Geometry: final body of the model. Coordinates: model frame, mm. Give positions to 0.01 mm unless a question says otherwise; leave off trailing zeros. Write each loop counter-clockwise with the first axis right and the second up, starting at its lowest first coordinate (ties: lowest second). Pieces come first, ordered by that corner, then holes. Notation, with made-up numbers: M -20,78 L 7,78 A35 ccw 7,114 Z; hole C 14,8.5 d11. An arc over 180 degrees is marked long. Use a Markdown table: item, result. Add a question column.
(1) Cut plane D-D (x = 0). Output: boundary loops of the cut face in (y, z) (3 decimals), plus the area to 3 significant figures.
(2) Material intervals for L1, parallel to X at y = -0.5, z = 4.25; L2, parallel to X at y = 5, z = 0.75; L3, parallel to X at y = -12, z = 4.75, sorted ascending.
(3) Cut plane A-A (x = -30.48). Output: boundary loops of the cut face in (y, z) (3 decimals), plus the area to 3 significant figures.
(4) Draft query along Y for faces 1 (the cylindrical face through (0.13, 15.11, 3.46)), 2 (the cylindrical face through (-45.713, 0.47, 3.461)), 3 (the cylindrical face through (19.98, 3.31, 3.44)), 4 (the cylindrical face through (-15.262, -10.234, 3.461)). Return one class per face: released by +Y, released by -Y, zero draft, split by the parting line, or undercut.
(5) Cut plane B-B (z = 3.75). Output: boundary loops of the cut face in (x, y) (3 decimals), plus the area to 3 significant figures.
(6) Cut plane C-C (y = -5). State how many separate pieces and enclosed holes the cut face has, plus the area to 3 significant figures.
(7) Pin query (flat end, axial travel): pin 1 Ø1 at (x, z) = (-11, 4) entering from -Y; pin 2 Ø1.5 at (x, z) = (-6, 4.5) entering from -Y. Return the tip coordinate at first contact, or that it passes through.
```python
from build123d import *

# Parameters (mm, degrees)
F0_R     = 11.0109
F1_DEPTH = 6.985
F2_SIZE  = 1.27
F3_SIZE  = 1.27


with BuildPart() as f1:
    # F0 (on Top) → F1 (new body)
    with BuildSketch(Plane.XY):
        with BuildLine():
            Line((15.1104870251, 0), (11.0109, 0))
            ThreePointArc((11.0109, 0), (0, -11.0109), (-11.0109, 0))
            Line((-11.0109, 0), (-15.1104870251, 0))
            ThreePointArc((-15.1104870251, 0), (-13.4476229912, -6.8911721805), (-8.8250173454, -12.2656384664))
            ThreePointArc((-8.8250173454, -12.2656384664), (0, -15.1104870251), (8.8250173454, -12.2656384664))
            ThreePointArc((8.8250173454, -12.2656384664), (13.4476229912, -6.8911721805), (15.1104870251, 0))
        make_face()
        with BuildLine():
            ThreePointArc((-11.0109, 0), (0, 11.0109), (11.0109, 0))
            Line((11.0109, 0), (15.1104870251, 0))
            ThreePointArc((15.1104870251, 0), (13.4476229912, 6.8911721805), (8.8250173454, 12.2656384664))
            ThreePointArc((8.8250173454, 12.2656384664), (0, 15.1104870251), (-8.8250173454, 12.2656384664))
            ThreePointArc((-8.8250173454, 12.2656384664), (-13.4476229912, 6.8911721805), (-15.1104870251, 0))
            Line((-15.1104870251, 0), (-11.0109, 0))
        make_face()
        with BuildLine():
            ThreePointArc((8.8250173454, 12.2656384664), (13.4476229912, 6.8911721805), (15.1104870251, 0))
            Line((15.1104870251, 0), (15.24, 0))
            ThreePointArc((15.24, 0), (16.8932840155, 6.9035316148), (21.4944289707, 12.3092287848))
            ThreePointArc((21.4944289707, 12.3092287848), (15.1667904983, 10.2333297341), (8.8250173454, 12.2656384664))
        make_face()
        with BuildLine():
            Line((15.24, 0), (15.1104870251, 0))
            ThreePointArc((15.1104870251, 0), (13.4476229912, -6.8911721805), (8.8250173454, -12.2656384664))
            ThreePointArc((8.8250173454, -12.2656384664), (15.1667904983, -10.2333297341), (21.4944289707, -12.3092287848))
            ThreePointArc((21.4944289707, -12.3092287848), (16.8932840155, -6.9035316148), (15.24, 0))
        make_face()
        with BuildLine():
            ThreePointArc((-8.8250173454, -12.2656384664), (-13.4476229912, -6.8911721805), (-15.1104870251, 0))
            Line((-15.1104870251, 0), (-15.24, 0))
            ThreePointArc((-15.24, 0), (-16.8932840155, -6.9035316148), (-21.4944289707, -12.3092287848))
            ThreePointArc((-21.4944289707, -12.3092287848), (-15.1667904983, -10.2333297341), (-8.8250173454, -12.2656384664))
        make_face()
        with BuildLine():
            Line((-15.24, 0), (-15.1104870251, 0))
            ThreePointArc((-15.1104870251, 0), (-13.4476229912, 6.8911721805), (-8.8250173454, 12.2656384664))
            ThreePointArc((-8.8250173454, 12.2656384664), (-15.1667904983, 10.2333297341), (-21.4944289707, 12.3092287848))
            ThreePointArc((-21.4944289707, 12.3092287848), (-16.8932840155, 6.9035316148), (-15.24, 0))
        make_face()
        with BuildLine():
            ThreePointArc((21.4944289707, 12.3092287848), (16.8932840155, 6.9035316148), (15.24, 0))
            ThreePointArc((15.24, 0), (16.8932840155, -6.9035316148), (21.4944289707, -12.3092287848))
            ThreePointArc((21.4944289707, -12.3092287848), (37.3835316148, -13.5867159845), (45.72, 0))
            ThreePointArc((45.72, 0), (37.3835316148, 13.5867159845), (21.4944289707, 12.3092287848))
        make_face()
        with BuildLine():
            ThreePointArc((41.4909, 0), (30.48, -11.0109), (19.4691, 0))
            ThreePointArc((19.4691, 0), (30.48, 11.0109), (41.4909, 0))
        make_face(mode=Mode.SUBTRACT)
        with BuildLine():
            ThreePointArc((-21.4944289707, -12.3092287848), (-16.8932840155, -6.9035316148), (-15.24, 0))
            ThreePointArc((-15.24, 0), (-16.8932840155, 6.9035316148), (-21.4944289707, 12.3092287848))
            ThreePointArc((-21.4944289707, 12.3092287848), (-45.72, 0), (-21.4944289707, -12.3092287848))
        make_face()
        with Locations((-30.48, 0)):
            Circle(F0_R, mode=Mode.SUBTRACT)
    extrude(amount=F1_DEPTH)

    # F2
    f2_edges = [f1.edges().sort_by_distance(p)[0] for p in [
        (-45.72, 0, 6.985),
    ]]
    chamfer(f2_edges, length=F2_SIZE)

    # F3
    f3_edges = [f1.edges().sort_by_distance(p)[0] for p in [
        (-45.72, 0, 0),
        (45.72, 0, 0),
        (0, -15.110487, 0),
        (15.16679, -10.23333, 0),
        (-15.16679, -10.23333, 0),
        (-15.16679, 10.23333, 0),
        (0, 15.110487, 0),
        (15.16679, 10.23333, 0),
    ]]
    chamfer(f3_edges, length=F3_SIZE)


solid = f1.part
```
Answer list:
| question | item | result |
|---|---|---|
| 1 | outline | M -15.11,1.27 L -13.84,0 L -11.011,0 L -11.011,6.985 L -13.84,6.985 L -15.11,5.715 Z; M 11.011,0 L 13.84,0 L 15.11,1.27 L 15.11,5.715 L 13.84,6.985 L 11.011,6.985 Z |
| 1 | area | 54.0 mm² |
| 2 | L1 | -45.71 to -41.48, -19.48 to -11, 11 to 19.48, 41.48 to 45.71 |
| 2 | L2 | -44.32 to -40.29, -20.67 to -9.81, 9.81 to 20.67, 40.29 to 44.32 |
| 2 | L3 | -39.87 to -21.05, -9.21 to 9.21, 21.05 to 39.87 |
| 3 | outline | M -15.24,1.27 L -13.97,0 L -11.011,0 L -11.011,6.985 L -13.97,6.985 L -15.24,5.715 Z; M 11.011,0 L 13.97,0 L 15.24,1.27 L 15.24,5.715 L 13.97,6.985 L 11.011,6.985 Z |
| 3 | area | 55.9 mm² |
| 4 | face 1 | released by +Y |
| 4 | face 2 | split by the parting line |
| 4 | face 3 | undercut |
| 4 | face 4 | released by -Y |
| 5 | outline | M -21.494,-12.309 A10.795 cw -8.825,-12.266 A15.11 ccw 8.825,-12.266 A10.795 cw 21.494,-12.309 A15.24 ccw long 21.494,12.309 A10.795 cw 8.825,12.266 A15.11 ccw -8.825,12.266 A10.795 cw -21.494,12.309 A15.24 ccw long Z; hole C -30.48,0 d22.022; hole C 0,0 d22.022; hole C 30.48,0 d22.022 |
| 5 | area | 1,150 mm² |
| 6 | separate pieces | 4 |
| 6 | enclosed holes | 0 |
| 6 | area | 212 mm² |
| 7 | pin 1 | y = -11.28 |
| 7 | pin 2 | y = -14.17 |
